Verification items for this drawing (mm, ordinates from the low corner). A direction names the side the tool comes from. Give positions to 0.01 mm unless a question says otherwise; leave off trailing zeros. Order: outer loops, then holes, each group sorted by start corner. A loop starts at its lowest first (then second) coordinate and runs counter-clockwise, first axis right, second up.
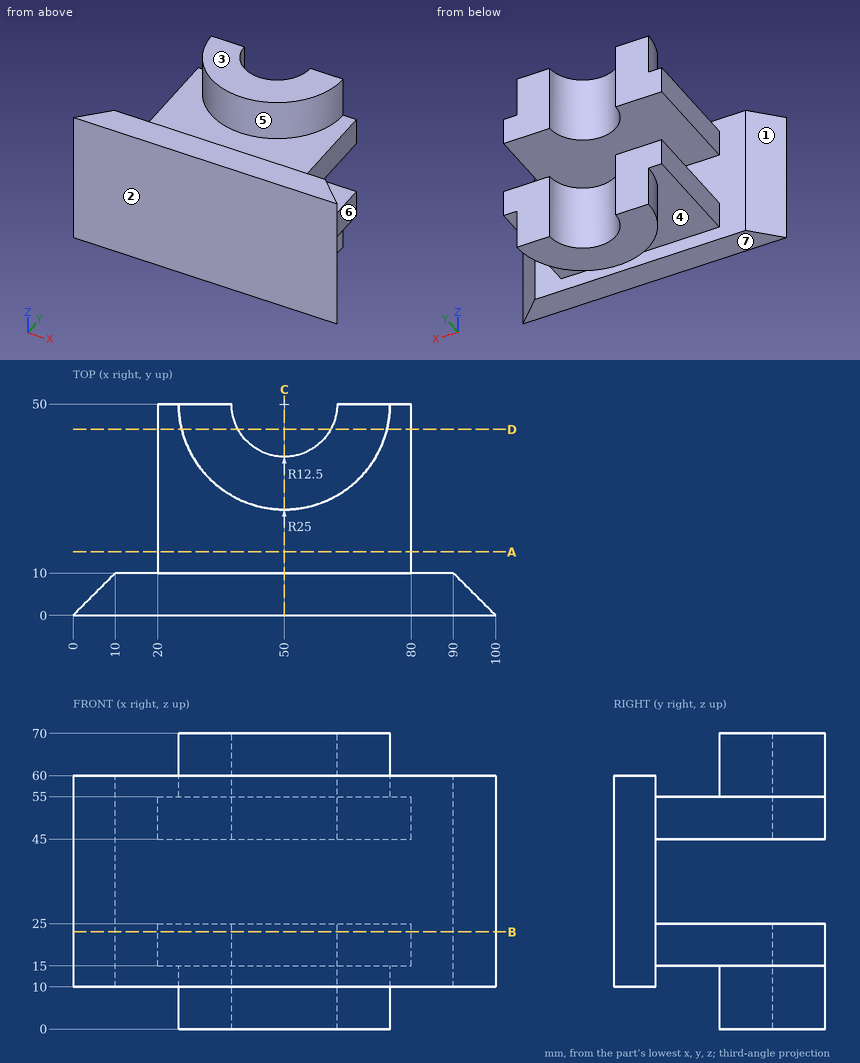
Q1. Release check for a two-part mould opening along Y. For the marked faces 1, 2, 3 and 4 record: pulls with the +Y half, pulls with the -Y half, needs draft (parallel to the pull), parting line crosses it, or undercut.
Q2. Cross-section at C-C, the plane x = 50. Record the boundary of the cut face in (y, z), and give its area (4 significant figures).
Q3. Gauge pin test, flat ends, axial feed: P1, Ø8, axis at x = 74.5, y = 3.5, coming from the -Z side; P2, Ø11, axis at y = 30, z = 52, coming from the +X side; P3, Ø3, axis at x = 43.5, y = 4.5, coming from the +Z side; P4, Ø2, axis at x = 81.5, y = 31, coming from the +Z side. Record the tip position at first contact, or that the pin passes through.
Q4. Access from +Z, -Z, +X, -X, +Y, -Y to the whole of each face (thin tool, end or side, straight path). Record for the marked faces 5, 6 and 7.
Q5. Thickness scan on L1, parallel to Z at x = 56, y = 12; L2, parallel to Y at x = 37.5, z = 32.5; L3, parallel to Z at x = 67, y = 7.5. Record the ranges inside material, lowest first.
Q6. Cross-section at A-A, the plane y = 15. Record the boundary of the cut face in (x, z), and give its area (3 significant figures).
Q7. Cross-section at D-D, the plane y = 44. Record the boundary of the cut face in (x, z), and give its area (3 significant figures).
Q8. Cross-section at B-B, the plane z = 23. Record the boundary of the cut face in (x, y), and give its area (3 significant figures).
Answers follow:
1. face 1: pulls with the +Y half
1. face 2: pulls with the -Y half
1. face 3: needs draft
1. face 4: undercut
2. outline: (0, 10) - (10, 10) - (10, 15) - (25, 15) - (25, 0) - (37.5, 0) - (37.5, 25) - (10, 25) - (10, 45) - (37.5, 45) - (37.5, 70) - (25, 70) - (25, 55) - (10, 55) - (10, 60) - (0, 60) - close
2. area: 1,425 mm2
3. P1: stops at z = 10
3. P2: stops at x = 80
3. P3: stops at z = 60
3. P4: passes through
4. face 5: +Z
4. face 6: +Z, -Z, +X, +Y
4. face 7: -Z, +X, -X, -Y
5. L1: z = 15 to 25, 45 to 55
5. L2: y = 0 to 10
5. L3: z = 10 to 60
6. outline: (20, 15) - (80, 15) - (80, 25) - (20, 25) - close; (20, 45) - (80, 45) - (80, 55) - (20, 55) - close
6. area: 1,200 mm2
7. outline: (20, 15) - (25.73, 15) - (25.73, 0) - (39.03, 0) - (39.03, 25) - (20, 25) - close; (20, 45) - (39.03, 45) - (39.03, 70) - (25.73, 70) - (25.73, 55) - (20, 55) - close; (60.97, 0) - (74.27, 0) - (74.27, 15) - (80, 15) - (80, 25) - (60.97, 25) - close; (60.97, 45) - (80, 45) - (80, 55) - (74.27, 55) - (74.27, 70) - (60.97, 70) - close
7. area: 1,560 mm2
8. outline: (0, 0) - (100, 0) - (90, 10) - (80, 10) - (80, 50) - (62.5, 50) arc R12.5 cw to (37.5, 50) - (20, 50) - (20, 10) - (10, 10) - close
8. area: 3,050 mm2
